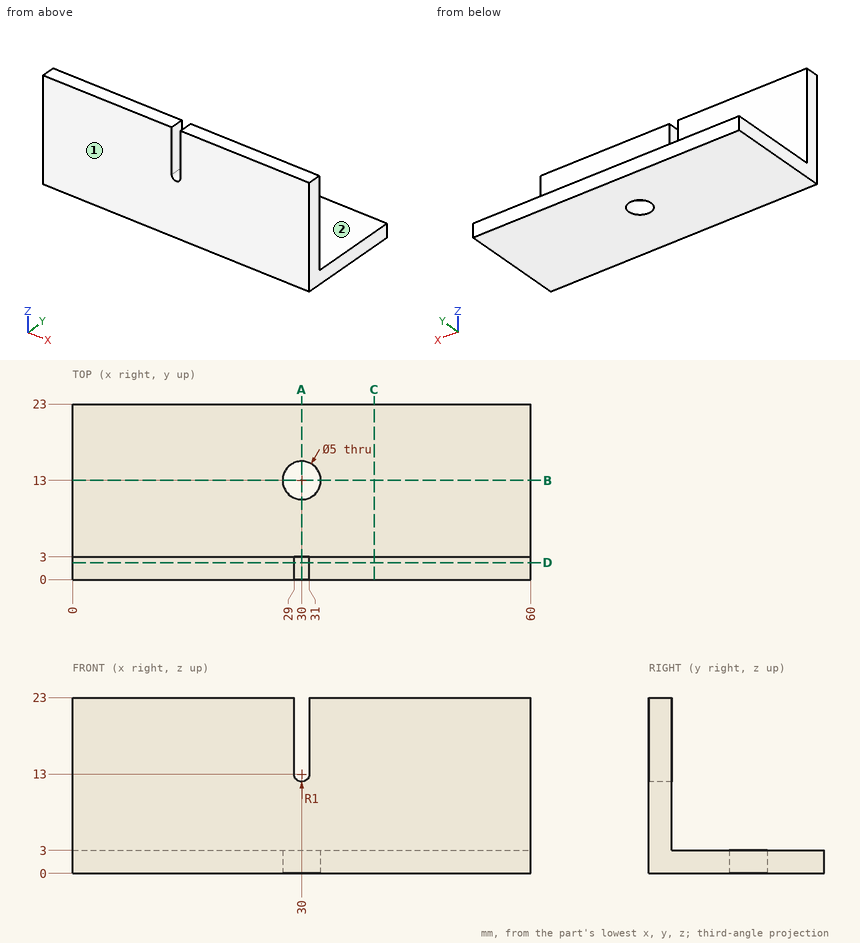
Geometry: see drawing. Coordinates: mm, zero at the bounding-box minimum. A direction names the side the tool comes from. Round coordinates to 2 decimals unless told otherwise and drop trailing zeros. Write each loop counter-clockwise with the first axis right and the second up, starting at its lowest first coordinate (ties: lowest second). Pieces come first, ordered by that corner, then holes. Notation, with made-up numbers: M 80.5,-4.5 L 138.5,-4.5 A22 ccw 138.5,24.5 Z; hole C 84.5,83.5 d7. An arc over 180 degrees is marked long. Answer as a JSON object with one key per item and string values. Group by question number.
(1) Reachability of the marked faces 1 and 2 from +Z, -Z, +X, -X, +Y, -Y: full face, straight path, thin tool, end or side. Return the list, or none.
(2) Section query B-B on y = 13. Output: boundary loops of the cut face in (x, z).
(3) Ray query, line 1 (Y direction, x = 30, z = 0.7); line 2 (Z direction, x = 35, y = 13). Return the intervals inside material, ascending. Write a range as [from, to].
(4) Section query C-C on x = 39.5. Output: boundary loops of the cut face in (y, z).
(5) First-contact query: pin 1 (2 mm diameter, centred on x = 35, y = 19.5, fed in from -Z); pin 2 (12 mm diameter, centred on x = 23.5, z = 16, fed in from +Y); pin 3 (6 mm diameter, centred on x = 43.5, y = 8.5, fed in from +Z). Flat tips, straight axial feed; report the tip coordinate or a pass-through.
(6) Section query A-A on x = 30. Output: boundary loops of the cut face in (y, z), then the cut area to 3 significant figures.
(7) Section query D-D on y = 2.25. Output: boundary loops of the cut face in (x, z), then the cut area to 3 significant figures.
Computed values:
{
 "1": {"face 1": "+Z, -Z, +X, -X, -Y", "face 2": "+Z, +X, -X, +Y"},
 "2": {"outline": "M 0,0 L 27.5,0 L 27.5,3 L 0,3 Z; M 32.5,0 L 60,0 L 60,3 L 32.5,3 Z"},
 "3": {"line 1": "[0, 10.5], [15.5, 23]", "line 2": "[0, 3]"},
 "4": {"outline": "M 0,0 L 23,0 L 23,3 L 3,3 L 3,23 L 0,23 Z"},
 "5": {"pin 1": "z = 0", "pin 2": "y = 3", "pin 3": "z = 3"},
 "6": {"outline": "M 0,0 L 10.5,0 L 10.5,3 L 3,3 L 3,12 L 0,12 Z; M 15.5,0 L 23,0 L 23,3 L 15.5,3 Z", "area": "81.0 mm^2"},
 "7": {"outline": "M 0,0 L 60,0 L 60,23 L 31,23 L 31,13 A1 cw 29,13 L 29,23 L 0,23 Z", "area": "1,360 mm^2"}
}
